Model file for the job. Use its own axes, mm. A direction names the side the tool comes from. Coordinates: 2 decimals unless noted, no trailing zeros. Write each loop counter-clockwise with the first axis right and the second up, starting at its lowest first coordinate (ties: lowest second). Pieces come first, ordered by that corner, then holes. Notation, with made-up numbers: M 60,37.5 L 75,37.5 A22 ccw 75,70.5 Z; hole C 14.5,-10 d10. An arc over 180 degrees is marked long. Put each result on its own line as item: value. Start each with the question number.
Q1. Pull direction X, two halves, no side cores. Call faces 6 (the flat face through (15, 7, 3)), 7 (the flat face through (-3.3, 0, 12.3)), 8 (the flat face through (-15, -9, 10)), 9 (the cylindrical face through (-19.524, 3.451, -4.336)): pulls with the +X half, pulls with the -X half, needs draft (parallel to the pull), parting line crosses it, or undercut.
Q2. Cut at D-D (z = 34). Write the cut outline in (x, y).
Q3. Drop flat-ended pins along their axis: pin 1 (3 mm diameter, centred on x = 32.5, y = -1.5, fed in from +Z); pin 2 (6 mm diameter, centred on x = 35, z = 0, fed in from +Y); pin 3 (8 mm diameter, centred on y = -6, z = 7, fed in from -X). Give the stop position or say it passes through.
Q4. Drill centre lines: line 1 along X through (y, z) = (-6.5, -14); line 2 along X through (y, z) = (-0.85, 0); line 3 along X through (y, z) = (5.5, 0). Where is each one in solid material? Low to high.
Q5. Cut at B-B (z = 0). Write the cut outline in (x, y), then the cut area to 4 significant figures.
Q6. Cut at C-C (x = 8.5). Write the cut outline in (y, z).
Q7. Cut at A-A (y = -2.25). Give the number of separate pieces and of enclosed holes in the cut face, then the cut area to 3 significant figures.
Q8. Which spindle directions (+Z, -Z, +X, -X, +Y, -Y) get a long thin tool onto all of the face, cutting with end or side? Do faces 1 (the flat face through (-32, -2, 5)), 2 (the flat face through (15, -9, 10)), 3 (the cylindrical face through (0.66, 3.451, -14.985)), 4 (the cylindrical face through (5.942, -5.895, -15.764)), 5 (the flat face through (30, -2, 24)). Say none if no direction does.
```python
from build123d import *

# Parameters (mm, degrees)
SKETCH_1_R          = 20
SKETCH_1_R_2        = 15
EXTRUDE_1_DEPTH     = 7
SKETCH_2_R          = 70
SKETCH_2_R_2        = 12.5
EXTRUDE_2_DEPTH     = 4
SKETCH_3_W          = 30
SKETCH_3_H          = 64
SKETCH_3_R          = 2
SKETCH_3_R_2        = 12.5
EXTRUDE_3_DEPTH     = 9.5
SKETCH_4_R          = 81.168465046
CUT_EXTRUDE_1_DEPTH = 9.5
CUT_EXTRUDE_START   = -15
SKETCH_6_R          = 2
CUT_EXTRUDE_2_DEPTH = 15
SKETCH_7_R          = 2.5
EXTRUDE_4_DEPTH     = 4


with BuildPart() as part:
    # Эскиз1 → Бобышка-Вытянуть1 (new body)
    with BuildSketch(Plane(origin=(0, 0, 0), x_dir=(1, 0, 0), z_dir=(0, 1, 0))):
        with Locations(Location((0, 0, 0), (0, 0, 270))):
            Circle(SKETCH_1_R)
        with Locations(Location((0, 0, 0), (0, 0, 270))):
            Circle(SKETCH_1_R_2, mode=Mode.SUBTRACT)
    extrude(amount=EXTRUDE_1_DEPTH)

    # Эскиз2 → Бобышка-Вытянуть2 (add)
    with BuildSketch(Plane.XZ):
        with Locations(Location((0, 0, 0), (0, 0, 270))):
            Circle(SKETCH_2_R)
        with Locations(Location((0, 0, 0), (0, 0, 270))):
            Circle(SKETCH_2_R_2, mode=Mode.SUBTRACT)
    extrude(amount=EXTRUDE_2_DEPTH)

    # Эскиз3 → Бобышка-Вытянуть3 (add)
    with BuildSketch(Plane.XZ.offset(4)):
        with Locations((0, 10)):
            Rectangle(SKETCH_3_W, SKETCH_3_H)
        with Locations(Location((-5, 34, 0), (0, 0, 270))):
            Circle(SKETCH_3_R, mode=Mode.SUBTRACT)
        with Locations(Location((5, 34, 0), (0, 0, 270))):
            Circle(SKETCH_3_R, mode=Mode.SUBTRACT)
        with Locations(Location((-5, -14, 0), (0, 0, 270))):
            Circle(SKETCH_3_R, mode=Mode.SUBTRACT)
        with Locations(Location((5, -14, 0), (0, 0, 270))):
            Circle(SKETCH_3_R, mode=Mode.SUBTRACT)
        with Locations(Location((0, 0, 0), (0, 0, 270))):
            Circle(SKETCH_3_R_2, mode=Mode.SUBTRACT)
    extrude(amount=EXTRUDE_3_DEPTH)

    # Эскиз4 → Вырез-Вытянуть1 (cut)
    with BuildSketch(Plane(origin=(0, 0, 0), x_dir=(1, 0, 0), z_dir=(0, 1, 0))):
        Circle(SKETCH_4_R)
        with BuildLine():
            Line((-30, 0), (-30, -42))
            Line((-30, -42), (30, -42))
            Line((30, -42), (30, 0))
            ThreePointArc((30, 0), (0, 30), (-30, 0))
        make_face(mode=Mode.SUBTRACT)
    extrude(amount=-CUT_EXTRUDE_1_DEPTH, mode=Mode.SUBTRACT)

    # Эскиз6 → Вырез-Вытянуть2 (cut)
    with BuildSketch(Plane.XZ.offset(13.5).offset(CUT_EXTRUDE_START)):
        with Locations(Location((-5, 34, 0), (0, 0, 270))):
            Circle(SKETCH_6_R)
        with Locations(Location((5, 34, 0), (0, 0, 270))):
            Circle(SKETCH_6_R)
        with Locations(Location((-5, -14, 0), (0, 0, 160.346175942))):
            Circle(SKETCH_6_R)
        with Locations(Location((5, -14, 0), (0, 0, 19.653824058))):
            Circle(SKETCH_6_R)
    extrude(amount=CUT_EXTRUDE_2_DEPTH, mode=Mode.SUBTRACT)

    # Эскиз7 → Бобышка-Вытянуть4 (add)
    # profile 1 of 3: a face of its own
    with BuildSketch(Plane(origin=(0, 0, 0), x_dir=(1, 0, 0), z_dir=(0, 1, 0))):
        with BuildLine():
            Line((-35, 5), (-27, 5))
            Line((-27, 5), (-27, -5))
            Line((-27, -5), (-35, -5))
            ThreePointArc((-35, -5), (-40, 0), (-35, 5))
        make_face()
        with Locations(Location((-35, 0, 0), (0, 0, 270))):
            Circle(SKETCH_7_R, mode=Mode.SUBTRACT)
    # profile 2 of 3: a face of its own
    with BuildSketch(Plane(origin=(0, 0, 0), x_dir=(1, 0, 0), z_dir=(0, 1, 0))):
        with BuildLine():
            Line((-5, 35), (-5, 27))
            Line((-5, 27), (5, 27))
            Line((5, 27), (5, 35))
            ThreePointArc((5, 35), (0, 40), (-5, 35))
        make_face()
        with Locations(Location((0, 35, 0), (0, 0, 270))):
            Circle(SKETCH_7_R, mode=Mode.SUBTRACT)
    # profile 3 of 3: a face of its own
    with BuildSketch(Plane(origin=(0, 0, 0), x_dir=(1, 0, 0), z_dir=(0, 1, 0))):
        with BuildLine():
            Line((35, 5), (27, 5))
            Line((27, 5), (27, -5))
            Line((27, -5), (35, -5))
            ThreePointArc((35, -5), (40, 0), (35, 5))
        make_face()
        with Locations(Location((35, 0, 0), (0, 0, 270))):
            Circle(SKETCH_7_R, mode=Mode.SUBTRACT)
    extrude(amount=-EXTRUDE_4_DEPTH)


solid = part.part
```
Computed values:
1. face 6: needs draft
1. face 7: undercut
1. face 8: pulls with the -X half
1. face 9: parting line crosses it
2. outline: M -30,-4 L -15,-4 L -15,-13.5 L -7,-13.5 L -7,0 L -30,0 Z; M -3,-13.5 L 3,-13.5 L 3,0 L -3,0 Z; M 7,-13.5 L 15,-13.5 L 15,-4 L 30,-4 L 30,0 L 7,0 Z
3. pin 1: z = 5
3. pin 2: y = 0
3. pin 3: x = -38.54
4. line 1: -15 to -7, -3 to 3, 7 to 15
4. line 2: -40 to -37.5, -32.5 to -12.5, 12.5 to 32.5, 37.5 to 40
4. line 3: -20 to -15, 15 to 20
5. outline: M -40,-4 L -37.5,-4 L -37.5,0 L -40,0 Z; M -32.5,-4 L -15,-4 L -15,-13.5 L -12.5,-13.5 L -12.5,0 L -15,0 L -15,7 L -20,7 L -20,0 L -32.5,0 Z; M 12.5,-13.5 L 15,-13.5 L 15,-4 L 32.5,-4 L 32.5,0 L 20,0 L 20,7 L 15,7 L 15,0 L 12.5,0 Z; M 37.5,-4 L 40,-4 L 40,0 L 37.5,0 Z
5. area: 297.5 mm2
6. outline: M -13.5,-22 L -4,-22 L -4,-28.77 L 0,-28.77 L 0,-18.1 L 7,-18.1 L 7,-12.36 L 0,-12.36 L 0,-9.17 L -13.5,-9.17 Z; M -13.5,9.17 L 0,9.17 L 0,12.36 L 7,12.36 L 7,18.1 L 0,18.1 L 0,42 L -13.5,42 Z
7. separate pieces: 1
7. enclosed holes: 8
7. area: 3,600 mm2
8. face 1: +Z, -X, +Y, -Y
8. face 2: +Z, -Z, +X, -Y
8. face 3: +Y
8. face 4: -Y
8. face 5: +Z, +X, +Y, -Y
